from build123d import *

# Parameters (mm, degrees)
BOSS_EXTRUDE1_DEPTH = 25
SKETCH2_R           = 1
SKETCH2_R_2         = 6
CUT_EXTRUDE1_DEPTH  = 58.3
FILLET2_R           = 2
SKETCH3_R           = 1.5
CUT_EXTRUDE2_DEPTH  = 42


with BuildPart() as part:
    # Sketch1 → Boss-Extrude1 (new body)
    with BuildSketch(Plane(origin=(0, 0, 0), x_dir=(1, 0, 0), z_dir=(0, 1, 0))):
        Polygon((-21.5, 0.5), (33.8, 0.5), (33.8, 40.5), (34.8, 40.5), (34.8, 0.5), (34.8, -0.5), (-22.5, -0.5), (-22.5, 0.5), (-22.5, 40.5), (-21.5, 40.5), align=None)
    extrude(amount=BOSS_EXTRUDE1_DEPTH)

    # Sketch2 → Cut-Extrude1 (cut, through all)
    with BuildSketch(Plane(origin=(34.8, 0, 0), x_dir=(0, 0, -1), z_dir=(1, 0, 0))):
        with Locations((28.5, 12.5)):
            Circle(SKETCH2_R)
        with Locations((38, 12.5)):
            Circle(SKETCH2_R_2)
        with Locations((31.282485579, 19.217514421)):
            Circle(SKETCH2_R)
        with Locations((38, 22)):
            Circle(SKETCH2_R)
        with Locations((38, 3)):
            Circle(SKETCH2_R)
        with Locations((31.282485579, 5.782485579)):
            Circle(SKETCH2_R)
    extrude(amount=-CUT_EXTRUDE1_DEPTH, mode=Mode.SUBTRACT)

    # Fillet2
    fillet2_edges = [part.edges().sort_by_distance(p)[0] for p in [
        (34.8, 12.5, 0.5),
        (-22.5, 12.5, 0.5),
        (-21.5, 12.5, -0.5),
        (33.8, 12.5, -0.5),
    ]]
    fillet(fillet2_edges, radius=FILLET2_R)

    # Sketch3 → Cut-Extrude2 (cut, through all)
    with BuildSketch(Plane.XY.offset(0.5)):
        with Locations((-10.85, 20)):
            Circle(SKETCH3_R)
        with Locations((23.15, 20)):
            Circle(SKETCH3_R)
        with Locations((-10.85, 5)):
            Circle(SKETCH3_R)
        with Locations((23.15, 5)):
            Circle(SKETCH3_R)
    extrude(amount=-CUT_EXTRUDE2_DEPTH, mode=Mode.SUBTRACT)


solid = part.part
Geometry: final body of the model. Coordinates: model frame, mm. A direction names the side the tool comes from. Give positions to 0.01 mm unless a question says otherwise; leave off trailing zeros. Order: outer loops, then holes, each group sorted by start corner. A loop starts at its lowest first (then second) coordinate and runs counter-clockwise, first axis right, second up. Notation, with made-up numbers: (-6, 43.5) -> (46, 43.5) arc R20 ccw to (46, 80.5) -> close; hole circle Ø5 at (-21.75, 29.25). An arc over 180 degrees is marked (long way). Answer as a JSON object with one key per item and string values.
Q1. Access query for faces 4 (the cylindrical face through (24.58, 5.45, 0.01)), 5 (the flat face through (6, 12, -0.5)). Directions: +Z, -Z, +X, -X, +Y, -Y. A direction counts if a zero-diameter tool reaches every point of the face in a straight line with its end or side. Return the directions, or none.
Entries:
{"face 4": "+Z, -Z", "face 5": "-Z, +Y, -Y"}
Q2. Draft query along Y for faces 1 (the cylindrical face through (-21.993, 12.668, -32.002)), 2 (the cylindrical face through (33.2, 12.68, -1.07)), 3 (the flat face through (19, 25, 0)). Return one class per face: released by +Y, released by -Y, zero draft, split by the parting line, or undercut.
Entries:
{"face 1": "undercut", "face 2": "zero draft", "face 3": "released by +Y"}
Q3. Material intervals for probe 1 along Y at (x, z) = (-21.9, -38); probe 2 along X at (y, z) = (23, -25.5); probe 3 along Z at (x, y) = (30.5, 2), sorted ascending.
Entries:
{"probe 1": "y = 0 to 2, 4 to 6.5, 18.5 to 21, 23 to 25", "probe 2": "x = -22.5 to -21.5, 33.8 to 34.8", "probe 3": "z = -0.5 to 0.5"}
Q4. Section B-B (z = -4). Output: boundary loops of the cut face in (x, y).
Entries:
{"outline": "(-22.5, 0) -> (-21.5, 0) -> (-21.5, 25) -> (-22.5, 25) -> close; (33.8, 0) -> (34.8, 0) -> (34.8, 25) -> (33.8, 25) -> close"}
Q5. Section D-D (z = -28.5). Output: boundary loops of the cut face in (x, y).
Entries:
{"outline": "(-22.5, 0) -> (-21.5, 0) -> (-21.5, 11.5) -> (-22.5, 11.5) -> close; (-22.5, 13.5) -> (-21.5, 13.5) -> (-21.5, 25) -> (-22.5, 25) -> close; (33.8, 0) -> (34.8, 0) -> (34.8, 11.5) -> (33.8, 11.5) -> close; (33.8, 13.5) -> (34.8, 13.5) -> (34.8, 25) -> (33.8, 25) -> close"}
Q6. Section C-C (y = 12.5). Output: boundary loops of the cut face in (x, z), plus the area to 3 significant figures.
Entries:
{"outline": "(-22.5, -32) -> (-21.5, -32) -> (-21.5, -29.5) -> (-22.5, -29.5) -> close; (-22.5, -27.5) -> (-21.5, -27.5) -> (-21.5, -2.5) arc R2 cw to (-19.5, -0.5) -> (31.8, -0.5) arc R2 cw to (33.8, -2.5) -> (33.8, -27.5) -> (34.8, -27.5) -> (34.8, -1.5) arc R2 ccw to (32.8, 0.5) -> (-20.5, 0.5) arc R2 ccw to (-22.5, -1.5) -> close; (33.8, -32) -> (34.8, -32) -> (34.8, -29.5) -> (33.8, -29.5) -> close", "area": "116 mm^2"}
Q7. Section A-A (x = -10.85). Output: boundary loops of the cut face in (y, z), plus the area to 3 significant figures.
Entries:
{"outline": "(0, -0.5) -> (3.5, -0.5) -> (3.5, 0.5) -> (0, 0.5) -> close; (6.5, -0.5) -> (18.5, -0.5) -> (18.5, 0.5) -> (6.5, 0.5) -> close; (21.5, -0.5) -> (25, -0.5) -> (25, 0.5) -> (21.5, 0.5) -> close", "area": "19.0 mm^2"}
Q8. First-contact query: pin 1 (2.5 mm diameter, centred on y = 3, z = -38, fed in from +X); pin 2 (5 mm diameter, centred on x = 23.15, y = 20, fed in from -Z). Flat tips, straight axial feed; report the tip coordinate or a pass-through.
Entries:
{"pin 1": "stops at x = 34.8", "pin 2": "stops at z = -0.5"}
